Input: part model. Units: mm. Frame: model coordinates. A direction names the side the tool comes from. Give positions to 0.01 mm unless a question says otherwise; leave off trailing zeros. Order: outer loops, then holes, each group sorted by start corner. A loop starts at its lowest first (then second) coordinate and runs counter-clockwise, first axis right, second up.
Autodesk Inventor part; units mm, degrees
ref_plane "YZ Plane" through (0, 0, 0) normal (1, 0, 0) x (0, 1, 0)
ref_plane "XZ Plane" through (0, 0, 0) normal (0, 1, 0) x (-1, 0, 0)
ref_plane "XY Plane" through (0, 0, 0) normal (0, 0, 1) x (1, 0, 0)
sketch "Sketch1" plane through (0, 0, 0) normal (0, 0, 1) x (1, 0, 0)
  line L0 (7.5, -28.5) -> (-7.5, -28.5)
  line L1 (-7.5, -28.5) -> (-7.5, 28.5)
  line L2 (-7.5, 28.5) -> (7.5, -28.5) construction
  line L3 (7.5, 28.5) -> (-7.5, -28.5) construction
  circle A0 centre (0, -20.5) radius 2.5
  line L4 (0, 24.5) -> (0, 11.5) construction
  line L5 (-2.5, 24.5) -> (-2.5, 11.5)
  line L6 (2.5, 11.5) -> (2.5, 24.5)
  arc A1 (2.5, 24.5) -> (-2.5, 24.5) centre (0, 24.5) ccw
  arc A2 (-2.5, 11.5) -> (2.5, 11.5) centre (0, 11.5) ccw
  line L7 (7.5, 31.5) -> (-7.5, 31.5)
  line L8 (-7.5, 31.5) -> (-7.5, -28.5)
  line L9 (7.5, 31.5) -> (7.5, -28.5)
  line L10 (7.5, -8.5) -> (7.5, -28.5)
  line L11 (7.5, -28.5) -> (22.5, -28.5)
  line L12 (22.5, -28.5) -> (22.5, -8.5)
  line L13 (22.5, -8.5) -> (7.5, -8.5)
  line L14 (7.5, -8.5) -> (7.5, -28.5)
  line L15 (22.5, -28.5) -> (24.5, -28.5)
  line L16 (24.5, -28.5) -> (24.5, -8.5)
  line L17 (24.5, -8.5) -> (22.5, -8.5)
  line L18 (22.5, -8.5) -> (22.5, -28.5)
  point P0 (0, 0)
  point P1 (0, 18)
  dimension "d7" = 15
  dimension "d8" = 57
  dimension "d9" = 5
  dimension "d10" = 13
  dimension "d11" = 5
  dimension "d12" = 60
  dimension "d39" = 15
  dimension "d40" = 20
  dimension "d41" = 2
extrude "Extrusion1" add sketch "Sketch1" along normal blind 2 contours L0 L1 L8 L7 L9
extrude "Extrusion2" add sketch "Sketch1" along normal blind 2 contours L9 L13 L12 L11 | L12 L17 L16 L15
extrude "Extrusion8" add sketch "Sketch1" against normal blind 60 contours L12 L17 L16 L15
sketch "Sketch6" plane through (-7.5, -28.5, 0) normal (0, -1, 0) x (1, 0, 0)
  line L0 (32, -60) -> (32, 2)
  line L1 (30, 0) -> (30, -60)
  line L2 (32, 2) -> (30, 2)
  line L3 (30, 2) -> (30, -60)
  line L4 (30, -60) -> (32, -60)
  line L5 (32, -60) -> (32, 2)
  line L6 (30, -60) -> (32, -60)
  line L7 (32, -60) -> (32, -20)
  line L8 (32, -20) -> (30, -20)
  line L9 (30, -20) -> (30, -60)
  point P0 (7.5, 0)
  dimension "d51" = 40
extrude "Extrusion9" cut sketch "Sketch6" against normal blind 20 contours L4 L1 L8 L0
extrude "Extrusion11" add sketch "Sketch6" along normal blind 20
sketch "Sketch8" plane through (24.5, -8.5, 2) normal (1, 0, 0) x (0, 0, -1)
  circle A0 centre (48, -30) radius 2.5
  point P0 (2, 8.5)
  dimension "d54" = 5
extrude "Extrusion12" cut sketch "Sketch8" against normal up to surface (2 mm away)
fillet "Fillet1" radius 3 10 edges at (23.5, -48.5, 2) (23.5, -8.5, -20) (23.5, -28.5, -20) (23.5, -28.5, -60) (23.5, -48.5, -60) (7.5, -8.5, 1) (22.5, -28.5, 1) (-7.5, -28.5, 1) (7.5, 31.5, 1) (-7.5, 31.5, 1)
properties part number "Rectangle_plate[1]"
1) Cut plane D-D (x = 15.5). Return the cut outline in (y, z).
2) Cut plane C-C (y = -17). Return the cut outline in (x, z).
3) Cut plane B-B (z = -46). Return the cut outline in (x, y).
4) Reachability of faces 1 (the face through (0, 9, 1)), 2 (the face through (23, -28.5, -40)), 3 (the face through (23, -8.5, -5)) from +Z, -Z, +X, -X, +Y, -Y: full face, straight path, thin tool, end or side. Return the list, or none.
5) Line query: probe 1 along Y at (x, z) = (0, 1.1); probe 2 along Y at (x, z) = (23.4, -46); probe 3 along Z at (x, y) = (-5, 1.5). Output: solid intervals per line, ascending.
6) Pull-direction query (X, two-part tool) for faces 4 (the face through (0, 27, 1)), 5 (the face through (6.64, 30.6, 1.01)), 6 (the face through (23.49, -47.64, 1.1)); classes: pulls with the +X half, pulls with the -X half, needs draft (parallel to the pull), parting line crosses it, or undercut.
7) Cut plane A-A (y = 13). Return the cut outline in (x, z).
8) First-contact query: P1, Ø8, axis at x = 0, y = -20.5, coming from the +Z side; P2, Ø9, axis at x = 3, y = 6, coming from the -Z side; P3, Ø1, axis at x = 2, z = 1.5, coming from the -Y side; P4, Ø20, axis at y = -29, z = -32, coming from the -X side. Flat tips, straight axial feed; report the tip coordinate or a pass-through.
Geometry says:
1. outline: (-28.5, 0) - (-8.5, 0) - (-8.5, 2) - (-28.5, 2) - close
2. outline: (-7.5, 0) - (22.5, 0) - (22.5, -20) - (24.5, -20) - (24.5, 2) - (-7.5, 2) - close
3. outline: (22.5, -48.5) - (24.5, -48.5) - (24.5, -41) - (22.5, -41) - close; (22.5, -36) - (24.5, -36) - (24.5, -28.5) - (22.5, -28.5) - close
4. face 1: +Z, -Z
4. face 2: -Z, +X, -X, +Y
4. face 3: +Z, -Z, +X, +Y
5. probe 1: y = -28.5 to -23, -18 to 9, 27 to 31.5
5. probe 2: y = -48.5 to -41, -36 to -28.5
5. probe 3: z = 0 to 2
6. face 4: undercut
6. face 5: pulls with the +X half
6. face 6: needs draft
7. outline: (-7.5, 0) - (-2.5, 0) - (-2.5, 2) - (-7.5, 2) - close; (2.5, 0) - (7.5, 0) - (7.5, 2) - (2.5, 2) - close
8. P1: stops at z = 2
8. P2: stops at z = 0
8. P3: stops at y = -28.5
8. P4: stops at x = 22.5
